from build123d import *

# Parameters (mm, degrees)
CROQUIS1_W              = 90.45
CROQUIS1_H              = 60
SALIENTE_EXTRUIR1_DEPTH = 2
CROQUIS2_W              = 90.45
CROQUIS2_H              = 60
CROQUIS2_W_2            = 87.55
CROQUIS2_H_2            = 57.1
SALIENTE_EXTRUIR2_DEPTH = 7
CROQUIS3_W              = 18.75
CROQUIS3_H              = 14.2
CORTAR_EXTRUIR1_DEPTH   = 9
CORTAR_EXTRUIR2_REACH   = 92.45
CROQUIS4_W              = 7
CROQUIS4_H              = 17
REDONDEO2_R             = 3
CROQUIS5_W              = 51.66
CROQUIS5_H              = 5.94
CORTAR_EXTRUIR3_DEPTH   = 2
CROQUIS6_W              = 6.3
CROQUIS6_H              = 21.36
CORTAR_EXTRUIR4_DEPTH   = 2
REDONDEO3_R             = 2
REDONDEO4_R             = 1
REDONDEO5_R             = 5


with BuildPart() as part:
    # Croquis1 → Saliente-Extruir1 (new body)
    with BuildSketch(Plane.XY):
        Rectangle(CROQUIS1_W, CROQUIS1_H)
    extrude(amount=-SALIENTE_EXTRUIR1_DEPTH)

    # Croquis2 → Saliente-Extruir2 (add)
    with BuildSketch(Plane.XY):
        Rectangle(CROQUIS2_W, CROQUIS2_H)
        Rectangle(CROQUIS2_W_2, CROQUIS2_H_2, mode=Mode.SUBTRACT)
    extrude(amount=SALIENTE_EXTRUIR2_DEPTH)

    # Croquis3 → Cortar-Extruir1 (cut)
    with BuildSketch(Plane(origin=(0, 0, -2), x_dir=(-1, 0, 0), z_dir=(0, 0, -1))):
        with Locations((-35.85, -18.95)):
            Rectangle(CROQUIS3_W, CROQUIS3_H)
        with Locations((-35.85, -0.95)):
            Rectangle(CROQUIS3_W, CROQUIS3_H)
    extrude(amount=-CORTAR_EXTRUIR1_DEPTH, mode=Mode.SUBTRACT)

    # Croquis4 → Cortar-Extruir2 (cut, up to next)
    with BuildSketch(Plane(origin=(45.225, 0, 0), x_dir=(0, 0, -1), z_dir=(1, 0, 0)), mode=Mode.PRIVATE) as cortar_extruir2_sk1:
        with Locations((-3.5, 17.75)):
            Rectangle(CROQUIS4_W, CROQUIS4_H)
    cortar_extruir2_tool1 = extrude(cortar_extruir2_sk1.sketch, amount=-CORTAR_EXTRUIR2_REACH, mode=Mode.PRIVATE) & part.part
    add(cortar_extruir2_tool1.solids().sort_by_distance((45.225, 17.75, 3.5))[0], mode=Mode.SUBTRACT)

    # Redondeo2
    redondeo2_edges = [part.edges().sort_by_distance(p)[0] for p in [
        (45.225, -30, 2.5),
        (-45.225, -30, 2.5),
        (-45.225, 30, 2.5),
        (45.225, 30, 2.5),
    ]]
    fillet(redondeo2_edges, radius=REDONDEO2_R)

    # Croquis5 → Cortar-Extruir3 (cut)
    with BuildSketch(Plane(origin=(0, 0, -2), x_dir=(-1, 0, 0), z_dir=(0, 0, -1))):
        with Locations((11.245, -24.58)):
            Rectangle(CROQUIS5_W, CROQUIS5_H)
    extrude(amount=-CORTAR_EXTRUIR3_DEPTH, mode=Mode.SUBTRACT)

    # Croquis6 → Cortar-Extruir4 (cut)
    with BuildSketch(Plane(origin=(0, 0, -2), x_dir=(-1, 0, 0), z_dir=(0, 0, -1))):
        with Locations((39.375, 0.11)):
            Rectangle(CROQUIS6_W, CROQUIS6_H)
        with Locations((-2.195, 17.77)):
            Rectangle(CROQUIS6_W, CROQUIS6_H)
    extrude(amount=-CORTAR_EXTRUIR4_DEPTH, mode=Mode.SUBTRACT)

    # Redondeo3
    redondeo3_edges = [part.edges().sort_by_distance(p)[0] for p in [
        (-36.225, -10.57, -1),
        (-36.225, 10.79, -1),
        (-42.525, 10.79, -1),
        (-42.525, -10.57, -1),
        (5.345, 7.09, -1),
        (5.345, 28.45, -1),
        (-0.955, 28.45, -1),
        (-0.955, 7.09, -1),
    ]]
    fillet(redondeo3_edges, radius=REDONDEO3_R)

    # Redondeo4
    redondeo4_edges = [part.edges().sort_by_distance(p)[0] for p in [
        (14.585, -27.55, -1),
        (14.585, -21.61, -1),
        (-37.075, -21.61, -1),
        (-37.075, -27.55, -1),
    ]]
    fillet(redondeo4_edges, radius=REDONDEO4_R)

    # Redondeo5
    redondeo5_edges = [part.edges().sort_by_distance(p)[0] for p in [
        (43.775, -9.95, 0),
        (43.775, 7.7, 0),
    ]]
    fillet(redondeo5_edges, radius=REDONDEO5_R)


solid = part.part
Here's how the part is built. I have some questions about the finished solid (model axes, mm). A direction names the side the tool comes from. Round coordinates to 2 decimals unless told otherwise and drop trailing zeros. Write each loop counter-clockwise with the first axis right and the second up, starting at its lowest first coordinate (ties: lowest second). Pieces come first, ordered by that corner, then holes. Notation, with made-up numbers: (76.5, 27.25) -> (107.5, 27.25) arc R23 ccw to (107.5, 46.25) -> close; hole circle Ø6 at (1.5, -22.5). An arc over 180 degrees is marked (long way). One line per item, written item: value.
1) For faces 1 (the face through (-44.37, -29.1, 2.56)), 2 (the face through (-36.225, 0, -1)), 3 (the face through (38, -8.05, -1)), 4 (the face through (-1, 0, -2)), 5 (the face through (-1, 28.55, 3)), which set-ups out of +Z, -Z, +X, -X, +Y, -Y let a thin tool reach every point of the face, with its end or its side?
Filled sheet:
face 1: +Z, -Z, -X, -Y
face 2: +Z, -Z
face 3: +Z, -Z, +X
face 4: -Z, +X, -X, +Y, -Y
face 5: +Z
2) Suppose I cut it at D-D on y = 12. List the corners of the cut face in (x, z) for me (3 decimals).
Filled sheet:
outline: (-45.225, -2) -> (-0.955, -2) -> (-0.955, 0) -> (-43.775, 0) -> (-43.775, 7) -> (-45.225, 7) -> close; (5.345, -2) -> (45.225, -2) -> (45.225, 0) -> (5.345, 0) -> close
3) I'm going to push flat-ended pins straight in: pin 1 Ø10 at (x, y) = (35, 2) entering from +Z; pin 2 Ø2 at (y, z) = (0.5, -1.5) entering from +X (3 decimals); pin 3 Ø4 at (y, z) = (1, 3) entering from +X (3 decimals). Where does each tip first touch, or does it pass through?
Filled sheet:
pin 1: stops at z = 0
pin 2: stops at x = 26.475
pin 3: stops at x = -43.775
4) We'd pull the mould along Y, two halves only. Please class faces 6 (the face through (5.345, 18, -1)), 7 (the face through (-44.37, 29.1, 2.44)), 8 (the face through (-1, -30, 2)), 9 (the face through (45.225, 14, -1)): released by +Y, released by -Y, zero draft, split by the parting line, or undercut.
Filled sheet:
face 6: undercut
face 7: released by +Y
face 8: released by -Y
face 9: zero draft
5) Suppose I cut it at A-A on x = -10. List the corners of the cut face in (y, z) for me, plus the area to 3 significant figures.
Filled sheet:
outline: (-30, -2) -> (-27.55, -2) -> (-27.55, 0) -> (-28.55, 0) -> (-28.55, 7) -> (-30, 7) -> close; (-21.61, -2) -> (30, -2) -> (30, 7) -> (28.55, 7) -> (28.55, 0) -> (-21.61, 0) -> close
area: 128 mm2
6) If I drill on line 1 (Y direction, x = -7, z = 3.75); line 2 (X direction, y = 6.5, z = 6.25) (3 decimals); line 3 (X direction, y = 20.5, z = 2.25) (3 decimals), over which ranges is the centre line in solid material (lowest first)? Write a range as [from, to].
Filled sheet:
line 1: y = [-30, -28.55], [28.55, 30]
line 2: x = [-45.225, -43.775], [43.775, 45.225]
line 3: x = [-45.225, -43.775]
7) Suppose I cut it at C-C on z = 2.25. List the corners of the cut face in (x, y) for me (3 decimals), plus the area to 3 significant figures.
Filled sheet:
outline: (-45.225, -27) arc R3 ccw to (-42.225, -30) -> (42.225, -30) arc R3 ccw to (45.225, -27) -> (45.225, -26.05) -> (43.775, -26.05) -> (43.775, -28.55) -> (-43.775, -28.55) -> (-43.775, 28.55) -> (43.775, 28.55) -> (43.775, 26.25) -> (45.225, 26.25) -> (45.225, 27) arc R3 ccw to (42.225, 30) -> (-42.225, 30) arc R3 ccw to (-45.225, 27) -> close; (42.951, -11.85) -> (45.225, -11.85) -> (45.225, -8.05) -> (42.951, -8.05) -> close; (42.951, 6.15) -> (45.225, 6.15) -> (45.225, 9.25) -> (42.951, 9.25) -> close
area: 360 mm2
8) Suppose I cut it at B-B on y = -5.5. List the corners of the cut face in (x, z) for me (3 decimals), plus the area to 3 significant figures.
Filled sheet:
outline: (-45.225, -2) -> (-42.525, -2) -> (-42.525, 0) -> (-43.775, 0) -> (-43.775, 7) -> (-45.225, 7) -> close; (-36.225, -2) -> (26.475, -2) -> (26.475, 0) -> (-36.225, 0) -> close
area: 141 mm2
